```python
from build123d import *

# Parameters (mm, degrees)
CHAMFER_1_SIZE           = 1.5
SKETCH_3_R               = 4
CUT_EXTRUDE_1_DEPTH      = 81.012499024
PATTERN_CIRCULAR_1_COUNT = 6
FILLET_1_R               = 2


with BuildPart() as part:
    # 草圖1 → 旋轉1 (revolve)
    with BuildSketch(Plane.XY, mode=Mode.PRIVATE) as revolve_1_sk:
        Polygon((0, 0), (0, 49), (7, 49), (7, 30), (19, 30), (19, 18.5), (22.5, 18.5), (22.5, 21), (47, 21), (47, 0), align=None)
    revolve(revolve_1_sk.sketch.rotate(Axis((0, 0, 0), (1, 0, 0)), 90), axis=Axis((0, 0, 0), (1, 0, 0)))

    # 草圖2 → 除料-旋轉1 (revolve, cut)
    with BuildSketch(Plane.XY, mode=Mode.PRIVATE) as cut_revolve_1_sk:
        Polygon((47, 0), (47, 10), (10, 10), (10, 22.5), (0, 22.5), (0, 0), align=None)
    revolve(cut_revolve_1_sk.sketch.rotate(Axis((0, 0, 0), (1, 0, 0)), 90), axis=Axis((0, 0, 0), (1, 0, 0)), mode=Mode.SUBTRACT)

    # 導角1
    chamfer_1_edges = [part.edges().sort_by_distance(p)[0] for p in [
        (47, 0, -21),
        (22.5, 0, -21),
    ]]
    chamfer(chamfer_1_edges, length=CHAMFER_1_SIZE)

    # 草圖3 → 伸長1 (cut, through all)
    with BuildSketch(Plane(origin=(7, 0, 0), x_dir=(0, 0, -1), z_dir=(1, 0, 0))):
        with Locations((0, 40)):
            Circle(SKETCH_3_R)
    cut_extrude_1 = extrude(amount=-CUT_EXTRUDE_1_DEPTH, mode=Mode.SUBTRACT)

    # 環狀複製排列1: 伸長1 ×6 about axis
    pattern_circular_1_axis = Axis((0, 0, 0), (1, 0, 0))
    for i in range(1, PATTERN_CIRCULAR_1_COUNT):
        add(cut_extrude_1.rotate(pattern_circular_1_axis, i * 360 / PATTERN_CIRCULAR_1_COUNT), mode=Mode.SUBTRACT)

    # 圓角1
    fillet_1_edges = [part.edges().sort_by_distance(p)[0] for p in [
        (7, 0, -49),
        (19, 0, -30),
        (7, 0, -30),
    ]]
    fillet(fillet_1_edges, radius=FILLET_1_R)


solid = part.part
```
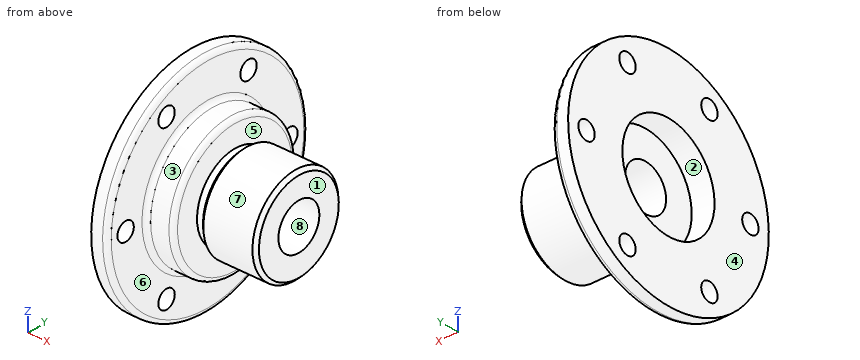
Can you work these out from the model? Positions are in its coordinate system, mm. Face numbers are marked on the shaded views. A direction names the side the tool comes from. Round coordinates to 2 decimals unless told otherwise and drop trailing zeros. Loops run counter-clockwise (first coordinate to the right, second up) from the corner with the lowest first, then second, coordinate; pieces in that order, holes last. Notation, with made-up numbers: M 83,17 L 128,17 A17 ccw 128,41 Z; hole C -32,39.5 d2. An arc over 180 degrees is marked long. Write item = value, one per line. Start each with the question number.
(1) Suppose I cut it at B-B on z = 0. Give the number of separate pieces and of enclosed holes in the cut face, plus the area to 3 significant figures.
(2) If we mould it in two halves opening along Z, with no side actions, what happens to the marked faces 6, 7 and 8? For each: released by +Z, released by -Z, zero draft, split by the parting line, or undercut.
(3) I need wall thicknesses on line 1 along Y through (x, z) = (4, 0); line 2 along Z through (x, y) = (9, 1); line 3 along Y through (x, z) = (29, 0). Which ranges of each line are inside material? Lowest first, please.
(4) Which directions (+Z, -Z, +X, -X, +Y, -Y) give clear straight access to the entire face, cutting with the end or side of a thin tool? Please do the marked faces 1, 2, 3, 4 and 5.
(5) Suppose I cut it at D-D on x = 15.5. Write out the boundary of the cut face in (y, z), plus the area to 3 significant figures.
(6) I'm going to push flat-ended pins straight in: P1, Ø13, axis at y = -40, z = 0, coming from the -X side; P2, Ø11.5, axis at y = 2.5, z = -6.5, coming from the -X side; P3, Ø8, axis at x = 26.5, z = 16.5, coming from the +Y side; P4, Ø13, axis at y = 20, z = 34.64, coming from the +X side. Where does each tip first touch, or does it pass through?
(7) Suppose I cut it at A-A on x = 37. Write out the boundary of the cut face in (y, z).
Answer block:
q1.separate_pieces = 4
q1.enclosed_holes = 0
q1.area = 1,260 mm²
q2.face_6 = zero draft
q2.face_7 = split by the parting line
q2.face_8 = undercut
q3.line_1 = -49 to -44, -36 to -22.5, 22.5 to 36, 44 to 49
q3.line_2 = -29.98 to -22.48, 22.48 to 29.98
q3.line_3 = -21 to -10, 10 to 21
q4.face_1 = +Z, -Z, +X, +Y, -Y
q4.face_2 = -X
q4.face_3 = +X
q4.face_4 = +Z, -Z, -X, +Y, -Y
q4.face_5 = none
q5.outline = C 0,0 d60; hole C 0,0 d20
q5.area = 2,510 mm²
q6.P1 = 0
q6.P2 = 10
q6.P3 = 16.87
q6.P4 = 7
q7.outline = C 0,0 d42; hole C 0,0 d20
